from build123d import *

# Parameters (mm, degrees)
SKETCH1_W           = 6
SKETCH1_H           = 4
BOSS_EXTRUDE1_DEPTH = 3
BOSS_EXTRUDE2_DEPTH = 2
CUT_EXTRUDE1_DEPTH  = 10


with BuildPart() as part:
    # Sketch1 → Boss-Extrude1 (new body)
    with BuildSketch(Plane(origin=(0, 0, 0), x_dir=(1, 0, 0), z_dir=(0, 1, 0))):
        with Locations((3, 2)):
            Rectangle(SKETCH1_W, SKETCH1_H)
    extrude(amount=BOSS_EXTRUDE1_DEPTH)

    # Sketch3 → Boss-Extrude2 (add)
    with BuildSketch(Plane(origin=(0, 3, 0), x_dir=(1, 0, 0), z_dir=(0, 1, 0))):
        Polygon((6, 4), (6, 0), (2, 4), align=None)
    extrude(amount=BOSS_EXTRUDE2_DEPTH)

    # Sketch4 → Cut-Extrude1 (cut)
    with BuildSketch(Plane(origin=(0, 3, 0), x_dir=(1, 0, 0), z_dir=(0, 1, 0))):
        Polygon((4, 0), (0, 4), (0, 0), align=None)
    extrude(amount=-CUT_EXTRUDE1_DEPTH, mode=Mode.SUBTRACT)


solid = part.part
Work out the finished part from the listing and answer in its coordinate system (mm). A direction names the side the tool comes from. Round coordinates to 2 decimals unless told otherwise and drop trailing zeros. Write each loop counter-clockwise with the first axis right and the second up, starting at its lowest first coordinate (ties: lowest second). Pieces come first, ordered by that corner, then holes. Notation, with made-up numbers: (-9.75, 44) -> (33.25, 44) arc R9 ccw to (33.25, 48) -> close; hole circle Ø1 at (28.5, 43). An arc over 180 degrees is marked (long way). Write each question's results on one line, items separated by ' | '.
Item 1: A cutting plane is placed at A-A, the plane z = -1.3. Determine the outline of the cut face in (x, y), plus the area to 3 significant figures.
Result set:
outline: (2.7, 0) -> (6, 0) -> (6, 5) -> (4.7, 5) -> (4.7, 3) -> (2.7, 3) -> close | area: 12.5 mm^2
Item 2: Find the intervals of material crossed by line 1 along Y through (x, z) = (3.25, -0.95); line 2 along Z through (x, y) = (5.5, 4.1); line 3 along X through (y, z) = (2.7, -1.95), in increasing order. Write a range as [from, to].
Result set:
line 1: [0, 3] | line 2: [-4, -0.5] | line 3: [2.05, 6]
Item 3: A cutting plane is placed at D-D, the plane x = 1.5. Determine the outline of the cut face in (y, z).
Result set:
outline: (0, -4) -> (3, -4) -> (3, -2.5) -> (0, -2.5) -> close
Item 4: A cutting plane is placed at C-C, the plane y = 2.6. Determine the outline of the cut face in (x, z).
Result set:
outline: (0, -4) -> (6, -4) -> (6, 0) -> (4, 0) -> close
Item 5: A flat-ended cylindrical pin translates along its axis: P1, Ø2, axis at x = 1.5, z = -2.5, coming from the +Y side. Find the tip coordinate at first contact, or state that the pin passes through.
Result set:
P1: y = 3
Item 6: Which of the six approach directions +Z, -Z, +X, -X, +Y, -Y give full straight-line access (tool end or side, diameter ignored) to faces 1 (the face through (4, 2, -4)), 2 (the face through (3, 3, -2))?
Result set:
face 1: -Z, +X, -X, +Y, -Y | face 2: +Z, -X, +Y
Item 7: A cutting plane is placed at B-B, the plane x = 3.5. Determine the outline of the cut face in (y, z).
Result set:
outline: (0, -4) -> (5, -4) -> (5, -2.5) -> (3, -2.5) -> (3, -0.5) -> (0, -0.5) -> close
